```python
from build123d import *

# Parameters (mm, degrees)
SKETCH2_W           = 240
SKETCH2_H           = 180
BOSS_EXTRUDE1_DEPTH = 100
SHELL1_T            = -10
FILLET3_R           = 10
FILLET4_R           = 10
SKETCH3_W           = 220
SKETCH3_H           = 90
CUT_EXTRUDE1_DEPTH  = 10
SKETCH6_W           = 69.206685732
SKETCH6_H           = 97.92746031
SKETCH6_W_2         = 62
SKETCH6_H_2         = 92
SKETCH6_W_3         = 84.432156592
SKETCH6_H_3         = 50.520880584
SKETCH6_W_4         = 76
SKETCH6_H_4         = 41
BOSS_EXTRUDE2_DEPTH = 5


with BuildPart() as part:
    # Sketch2 → Boss-Extrude1 (new body)
    with BuildSketch(Plane(origin=(0, 0, 0), x_dir=(1, 0, 0), z_dir=(0, 1, 0))):
        with Locations((91.04519774, -71.073446328)):
            Rectangle(SKETCH2_W, SKETCH2_H)
    extrude(amount=BOSS_EXTRUDE1_DEPTH)

    # Shell1
    shell1_openings = [part.faces().sort_by_distance(p)[0] for p in [
        (91.04519774, 100, 71.073446328),
    ]]
    offset(amount=SHELL1_T, openings=shell1_openings, kind=Kind.INTERSECTION)

    # Fillet3
    fillet3_edges = [part.edges().sort_by_distance(p)[0] for p in [
        (-28.95480226, 50, -18.926553672),
        (211.04519774, 50, -18.926553672),
        (211.04519774, 50, 161.073446328),
        (-28.95480226, 50, 161.073446328),
    ]]
    fillet(fillet3_edges, radius=FILLET3_R)

    # Fillet4
    fillet4_edges = [part.edges().sort_by_distance(p)[0] for p in [
        (-28.95480226, 0, 71.073446328),
        (91.04519774, 0, -18.926553672),
        (211.04519774, 0, 71.073446328),
        (91.04519774, 0, 161.073446328),
        (208.116265552, 0, 158.14451414),
        (208.116265552, 0, -15.997621484),
        (-26.025870072, 0, 158.14451414),
        (-26.025870072, 0, -15.997621484),
    ]]
    fillet(fillet4_edges, radius=FILLET4_R)

    # Sketch3 → Cut-Extrude1 (cut)
    with BuildSketch(Plane(origin=(0, 0, -18.926553672), x_dir=(-1, 0, 0), z_dir=(0, 0, -1))):
        with Locations((-91.04519774, 55)):
            Rectangle(SKETCH3_W, SKETCH3_H)
    extrude(amount=-CUT_EXTRUDE1_DEPTH, mode=Mode.SUBTRACT)

    # Sketch6 → Boss-Extrude2 (add)
    # profile 1 of 2: a face of its own
    with BuildSketch(Plane(origin=(0, 10, 0), x_dir=(1, 0, 0), z_dir=(0, 1, 0))):
        with Locations((32.200405027, -65.396277703)):
            Rectangle(SKETCH6_W, SKETCH6_H)
        with Locations((32.04519774, -65.073446328)):
            Rectangle(SKETCH6_W_2, SKETCH6_H_2, mode=Mode.SUBTRACT)
    # profile 2 of 2: a face of its own
    with BuildSketch(Plane(origin=(0, 10, 0), x_dir=(1, 0, 0), z_dir=(0, 1, 0))):
        with Locations((152.6200382, -98.44247014)):
            Rectangle(SKETCH6_W_3, SKETCH6_H_3)
        with Locations((152.556361047, -98.18046442)):
            Rectangle(SKETCH6_W_4, SKETCH6_H_4, mode=Mode.SUBTRACT)
    extrude(amount=BOSS_EXTRUDE2_DEPTH)


solid = part.part
```
Check sheet for the modelled part. Datum: model origin and axes. Units: mm. A direction names the side the tool comes from. Round coordinates to 2 decimals unless told otherwise and drop trailing zeros. Loops run counter-clockwise (first coordinate to the right, second up) from the corner with the lowest first, then second, coordinate; pieces in that order, holes last. Notation, with made-up numbers: (84, 79) -> (128, 79) arc R14 ccw to (128, 87) -> close; hole circle Ø3 at (-10.75, 69.5). An arc over 180 degrees is marked (long way). Answer in a Markdown table with one row per item.
Q1. Sectioned sample at B-B on x = 20.5. Enter the section's corners in (y, z), then the cut area to 3 significant figures.
Data:
| item | result |
|---|---|
| outline | (0, -8.93) arc R10 ccw to (10, -18.93) -> (10, 16.43) -> (15, 16.43) -> (15, 19.07) -> (10, 19.07) -> (10, 111.07) -> (15, 111.07) -> (15, 114.36) -> (10, 114.36) -> (10, 151.07) -> (100, 151.07) -> (100, 161.07) -> (10, 161.07) arc R10 ccw to (0, 151.07) -> close |
| area | 2,690 mm^2 |
Q2. Go/stop test with flat-tipped pins: P1, Ø5, axis at x = 185, y = 33.5, coming from the -Z side; P2, Ø1.5, axis at x = 36, y = 12, coming from the -Z side; P3, Ø20.5, axis at x = 165, z = 104, coming from the +Y side. Record where each tip stops, or that it passes through.
Data:
| item | result |
|---|---|
| P1 | stops at z = 151.07 |
| P2 | stops at z = 16.43 |
| P3 | stops at y = 10 |
Q3. Sectioned sample at A-A on y = 68. Enter the section's corners in (x, z), then the cut area to 3 significant figures.
Data:
| item | result |
|---|---|
| outline | (-28.95, -8.93) arc R10 ccw to (-18.95, -18.93) -> (-18.95, 151.07) -> (201.05, 151.07) -> (201.05, -18.93) arc R10 ccw to (211.05, -8.93) -> (211.05, 151.07) arc R10 ccw to (201.05, 161.07) -> (-18.95, 161.07) arc R10 ccw to (-28.95, 151.07) -> close |
| area | 5,710 mm^2 |
Q4. Thickness scan on L1, parallel to Z at x = 172.5, y = 11; L2, parallel to X at y = 73.5, z = 87.5; L3, parallel to Y at x = -3.5, z = 88.5. Record the ranges inside material, lowest first.
Data:
| item | result |
|---|---|
| L1 | z = 73.18 to 77.68, 118.68 to 123.7, 151.07 to 161.07 |
| L2 | x = -28.95 to -18.95, 201.05 to 211.05 |
| L3 | y = 0 to 10 |
Q5. Sectioned sample at C-C on z = -3. Enter the section's corners in (x, y).
Data:
| item | result |
|---|---|
| outline | (-28.95, 10) arc R10 ccw to (-18.95, 0) -> (201.05, 0) arc R10 ccw to (211.05, 10) -> (211.05, 100) -> (201.05, 100) -> (201.05, 10) -> (-18.95, 10) -> (-18.95, 100) -> (-28.95, 100) -> close |
Q6. Sectioned sample at D-D on x = 186. Enter the section's corners in (y, z), then the cut area to 3 significant figures.
Data:
| item | result |
|---|---|
| outline | (0, -8.93) arc R10 ccw to (10, -18.93) -> (10, 73.18) -> (15, 73.18) -> (15, 77.68) -> (10, 77.68) -> (10, 118.68) -> (15, 118.68) -> (15, 123.7) -> (10, 123.7) -> (10, 151.07) -> (100, 151.07) -> (100, 161.07) -> (10, 161.07) arc R10 ccw to (0, 151.07) -> close |
| area | 2,700 mm^2 |
Q7. Release check for a two-part mould opening along X. For faces 4 (the face through (-2.403, 12, 66)), 5 (the face through (-26.1, 55.63, 158.07)), 6 (the face through (90, 0, 70)) record: released by +X, released by -X, zero draft, split by the parting line, or undercut.
Data:
| item | result |
|---|---|
| face 4 | undercut |
| face 5 | released by -X |
| face 6 | zero draft |
Q8. Set-up check for faces 1 (the face through (110.404, 12, 99)), 2 (the face through (114.556, 12, 98)), 3 (the face through (208.194, 3.007, 72.193)): record each of +Z, -Z, +X, -X, +Y, -Y from which the full face is reachable in a straight line by a thin tool's end or side.
Data:
| item | result |
|---|---|
| face 1 | -Z, +Y |
| face 2 | +Y |
| face 3 | +Z, -Z, +X, -Y |
